```python
from build123d import *

# Parameters (mm, degrees)
CROQUIS1_R                  = 3.1
SALIENTE_EXTRUIR1_DEPTH     = 2.5
CROQUIS2_W                  = 6.5
CROQUIS2_H                  = 10
SALIENTE_EXTRUIR3_DEPTH     = 6
CROQUIS5_W                  = 1.5
CROQUIS5_H                  = 10
CORTAR_EXTRUIR2_DEPTH       = 3
SALIENTE_EXTRUIR4_START     = -3
CROQUIS6_W                  = 5
CROQUIS6_H                  = 10
SALIENTE_EXTRUIR4_DEPTH     = 4
REDONDEO1_R                 = 3
CROQUIS7_W                  = 6.5
CROQUIS7_H                  = 10
SALIENTE_EXTRUIR5_DEPTH     = 3
CHAFL_N1_SIZE2              = 3
CHAFL_N1_SIZE               = 1.732050808
CROQUIS8_W                  = 5
CROQUIS8_H                  = 10
SALIENTE_EXTRUIR6_DEPTH     = 3
CROQUIS9_W                  = 6.5
CROQUIS9_H                  = 10
SALIENTE_EXTRUIR7_DEPTH     = 3
REDONDEO2_R                 = 3
CHAFL_N2_SIZE2              = 3
CHAFL_N2_SIZE               = 1.732050808
REDONDEO1_OF_SIMETR_A1_R    = 3
CHAFL_N1_OF_SIMETR_A1_SIZE2 = 1.732050808
CHAFL_N1_OF_SIMETR_A1_SIZE  = 3
REDONDEO2_OF_SIMETR_A1_R    = 3
CHAFL_N2_OF_SIMETR_A1_SIZE2 = 1.732050808
CHAFL_N2_OF_SIMETR_A1_SIZE  = 3
CROQUIS10_W                 = 10
CROQUIS10_H                 = 6.5
SALIENTE_EXTRUIR9_DEPTH     = 6
CROQUIS12_W                 = 10
CROQUIS12_H                 = 1.5
CORTAR_EXTRUIR6_DEPTH       = 3
CROQUIS13_W                 = 10
CROQUIS13_H                 = 5
SALIENTE_EXTRUIR10_DEPTH    = 3
CROQUIS14_W                 = 10
CROQUIS14_H                 = 6.5
SALIENTE_EXTRUIR11_DEPTH    = 3
REDONDEO3_R                 = 3
CHAFL_N3_SIZE2              = 1.732050808
CHAFL_N3_SIZE               = 3
REDONDEO3_OF_SIMETR_A2_R    = 3
CHAFL_N3_OF_SIMETR_A2_SIZE2 = 3
CHAFL_N3_OF_SIMETR_A2_SIZE  = 1.732050808
SIMETR_A3_START             = 26.922069807
SIMETR_A3_DEPTH             = 10


# Read off the part's stored shape, not the designer's step: Simetría3
with BuildPart() as part:
    # Croquis1 → Saliente-Extruir1 (new body)
    with BuildSketch(Plane.XY):
        with BuildLine():
            Line((32.732069807, -35), (16.823581959, -35))
            Line((16.823581959, -35), (16.823581959, -55))
            Line((16.823581959, -55), (42.732069807, -55))
            ThreePointArc((42.732069807, -55), (56.874205431, -49.142135624), (62.732069807, -35))
            Line((62.732069807, -35), (62.732069807, 35))
            ThreePointArc((62.732069807, 35), (56.874205431, 49.142135624), (42.732069807, 55))
            Line((42.732069807, 55), (18.885856119, 55))
            Line((18.885856119, 55), (18.885856119, 45))
            Line((18.885856119, 45), (-9.114143881, 45))
            Line((-9.114143881, 45), (-9.114143881, 55))
            Line((-9.114143881, 55), (-32.96035757, 55))
            ThreePointArc((-32.96035757, 55), (-47.102493193, 49.142135624), (-52.96035757, 35))
            Line((-52.96035757, 35), (-52.96035757, -35))
            ThreePointArc((-52.96035757, -35), (-47.102493193, -49.142135624), (-32.96035757, -55))
            Line((-32.96035757, -55), (-6.267930193, -55))
            Line((-6.267930193, -55), (-6.267930193, -35))
            Line((-6.267930193, -35), (-22.96035757, -35))
            ThreePointArc((-22.96035757, -35), (-30.031425382, -32.071067812), (-32.96035757, -25))
            Line((-32.96035757, -25), (-32.96035757, 15.854777846))
            ThreePointArc((-32.96035757, 15.854777846), (-29.16035757, 20.3), (-32.96035757, 24.745222154))
            Line((-32.96035757, 24.745222154), (-32.96035757, 25))
            ThreePointArc((-32.96035757, 25), (-30.031425382, 32.071067812), (-22.96035757, 35))
            Line((-22.96035757, 35), (32.732069807, 35))
            ThreePointArc((32.732069807, 35), (39.803137619, 32.071067812), (42.732069807, 25))
            Line((42.732069807, 25), (42.732069807, 24.745222154))
            ThreePointArc((42.732069807, 24.745222154), (38.932069807, 20.3), (42.732069807, 15.854777846))
            Line((42.732069807, 15.854777846), (42.732069807, -25))
            ThreePointArc((42.732069807, -25), (39.803137619, -32.071067812), (32.732069807, -35))
        make_face()
        with Locations((20.823581959, -39.7)):
            Circle(CROQUIS1_R, mode=Mode.SUBTRACT)
        with Locations((-10.267930193, -39.7)):
            Circle(CROQUIS1_R, mode=Mode.SUBTRACT)
        with Locations((43.432069807, 20.3)):
            Circle(CROQUIS1_R, mode=Mode.SUBTRACT)
        with Locations((-33.66035757, 20.3)):
            Circle(CROQUIS1_R, mode=Mode.SUBTRACT)
    extrude(amount=SALIENTE_EXTRUIR1_DEPTH)

    # Croquis2 → Saliente-Extruir3 (add)
    with BuildSketch(Plane(origin=(0, 0, 0), x_dir=(-1, 0, 0), z_dir=(0, 0, -1))):
        with Locations((41.71035757, -20)):
            Rectangle(CROQUIS2_W, CROQUIS2_H)
        with Locations((41.71035757, 20)):
            Rectangle(CROQUIS2_W, CROQUIS2_H)
    saliente_extruir3 = extrude(amount=SALIENTE_EXTRUIR3_DEPTH)

    # Croquis5 → Cortar-Extruir2 (cut)
    with BuildSketch(Plane(origin=(0, 0, 0), x_dir=(-1, 0, 0), z_dir=(0, 0, -1))):
        with Locations((39.21035757, -20)):
            Rectangle(CROQUIS5_W, CROQUIS5_H)
        with Locations((39.21035757, 20)):
            Rectangle(CROQUIS5_W, CROQUIS5_H)
    cortar_extruir2 = extrude(amount=CORTAR_EXTRUIR2_DEPTH, mode=Mode.SUBTRACT)

    # Croquis6 → Saliente-Extruir4 (add)
    with BuildSketch(Plane(origin=(-38.46035757, 25, -6), x_dir=(1, 0, 0), z_dir=(0, 0, 1)).offset(SALIENTE_EXTRUIR4_START)):
        with Locations((-4, -5)):
            Rectangle(CROQUIS6_W, CROQUIS6_H)
    saliente_extruir4 = extrude(amount=SALIENTE_EXTRUIR4_DEPTH)

    # Redondeo1
    redondeo1_edges = [part.edges().sort_by_distance(p)[0] for p in [
        (-44.96035757, 20, 0),
    ]]
    fillet(redondeo1_edges, radius=REDONDEO1_R)

    # Croquis7 → Saliente-Extruir5 (add)
    with BuildSketch(Plane(origin=(0, 0, -9), x_dir=(-1, 0, 0), z_dir=(0, 0, -1))):
        with Locations((41.71035757, 20)):
            Rectangle(CROQUIS7_W, CROQUIS7_H)
    saliente_extruir5 = extrude(amount=SALIENTE_EXTRUIR5_DEPTH)

    # Chaflán1
    chafl_n1_edges = [part.edges().sort_by_distance(p)[0] for p in [
        (-38.46035757, 20, -12),
    ]]
    chafl_n1_side = [part.faces().sort_by_distance(p)[0] for p in [
        (-38.494998586, 20, -12),
    ]]
    chamfer(chafl_n1_edges, length=CHAFL_N1_SIZE - 0.0001, length2=CHAFL_N1_SIZE2 - 0.0001, reference=chafl_n1_side[0])  # a hair under: the kernel refuses the full size

    # Croquis8 → Saliente-Extruir6 (add)
    with BuildSketch(Plane(origin=(0, 0, -6), x_dir=(-1, 0, 0), z_dir=(0, 0, -1))):
        with Locations((42.46035757, -20)):
            Rectangle(CROQUIS8_W, CROQUIS8_H)
    saliente_extruir6 = extrude(amount=SALIENTE_EXTRUIR6_DEPTH)

    # Croquis9 → Saliente-Extruir7 (add)
    with BuildSketch(Plane(origin=(0, 0, -9), x_dir=(-1, 0, 0), z_dir=(0, 0, -1))):
        with Locations((41.71035757, -20)):
            Rectangle(CROQUIS9_W, CROQUIS9_H)
    saliente_extruir7 = extrude(amount=SALIENTE_EXTRUIR7_DEPTH)

    # Redondeo2
    redondeo2_edges = [part.edges().sort_by_distance(p)[0] for p in [
        (-44.96035757, -20, 0),
    ]]
    fillet(redondeo2_edges, radius=REDONDEO2_R)

    # Chaflán2
    chafl_n2_edges = [part.edges().sort_by_distance(p)[0] for p in [
        (-38.46035757, -20, -12),
    ]]
    chafl_n2_side = [part.faces().sort_by_distance(p)[0] for p in [
        (-38.494998586, -20, -12),
    ]]
    chamfer(chafl_n2_edges, length=CHAFL_N2_SIZE - 0.0001, length2=CHAFL_N2_SIZE2 - 0.0001, reference=chafl_n2_side[0])  # a hair under: the kernel refuses the full size

    # Simetría1: Saliente-Extruir3, Cortar-Extruir2, Saliente-Extruir4, Saliente-Extruir5, Saliente-Extruir6, Saliente-Extruir7 across plane
    add(saliente_extruir3.mirror(Plane(origin=(5.277069807, 0, 0), x_dir=(0, 0, 1), z_dir=(1, 0, 0))))
    add(cortar_extruir2.mirror(Plane(origin=(5.277069807, 0, 0), x_dir=(0, 0, 1), z_dir=(1, 0, 0))), mode=Mode.SUBTRACT)
    add(saliente_extruir4.mirror(Plane(origin=(5.277069807, 0, 0), x_dir=(0, 0, 1), z_dir=(1, 0, 0))))
    add(saliente_extruir5.mirror(Plane(origin=(5.277069807, 0, 0), x_dir=(0, 0, 1), z_dir=(1, 0, 0))))
    add(saliente_extruir6.mirror(Plane(origin=(5.277069807, 0, 0), x_dir=(0, 0, 1), z_dir=(1, 0, 0))))
    add(saliente_extruir7.mirror(Plane(origin=(5.277069807, 0, 0), x_dir=(0, 0, 1), z_dir=(1, 0, 0))))

    # Redondeo1 of Simetría1
    redondeo1_of_simetr_a1_edges = [part.edges().sort_by_distance(p)[0] for p in [
        (55.514497184, 20, 0),
    ]]
    fillet(redondeo1_of_simetr_a1_edges, radius=REDONDEO1_OF_SIMETR_A1_R)

    # Chaflán1 of Simetría1
    chafl_n1_of_simetr_a1_edges = [part.edges().sort_by_distance(p)[0] for p in [
        (49.014497184, 20, -12),
    ]]
    chafl_n1_of_simetr_a1_side = [part.faces().sort_by_distance(p)[0] for p in [
        (49.014497184, 20, -11.965358984),
    ]]
    chamfer(chafl_n1_of_simetr_a1_edges, length=CHAFL_N1_OF_SIMETR_A1_SIZE - 0.0001, length2=CHAFL_N1_OF_SIMETR_A1_SIZE2 - 0.0001, reference=chafl_n1_of_simetr_a1_side[0])  # a hair under: the kernel refuses the full size

    # Redondeo2 of Simetría1
    redondeo2_of_simetr_a1_edges = [part.edges().sort_by_distance(p)[0] for p in [
        (55.514497184, -20, 0),
    ]]
    fillet(redondeo2_of_simetr_a1_edges, radius=REDONDEO2_OF_SIMETR_A1_R)

    # Chaflán2 of Simetría1
    chafl_n2_of_simetr_a1_edges = [part.edges().sort_by_distance(p)[0] for p in [
        (49.014497184, -20, -12),
    ]]
    chafl_n2_of_simetr_a1_side = [part.faces().sort_by_distance(p)[0] for p in [
        (49.014497184, -20, -11.965358984),
    ]]
    chamfer(chafl_n2_of_simetr_a1_edges, length=CHAFL_N2_OF_SIMETR_A1_SIZE - 0.0001, length2=CHAFL_N2_OF_SIMETR_A1_SIZE2 - 0.0001, reference=chafl_n2_of_simetr_a1_side[0])  # a hair under: the kernel refuses the full size

    # Croquis10 → Saliente-Extruir9 (add)
    with BuildSketch(Plane(origin=(0, 0, 0), x_dir=(-1, 0, 0), z_dir=(0, 0, -1))):
        with Locations((21.367930193, -46.75)):
            Rectangle(CROQUIS10_W, CROQUIS10_H)
    saliente_extruir9 = extrude(amount=SALIENTE_EXTRUIR9_DEPTH)

    # Croquis12 → Cortar-Extruir6 (cut)
    with BuildSketch(Plane(origin=(0, 0, 0), x_dir=(-1, 0, 0), z_dir=(0, 0, -1))):
        with Locations((21.367930193, -44.25)):
            Rectangle(CROQUIS12_W, CROQUIS12_H)
    cortar_extruir6 = extrude(amount=CORTAR_EXTRUIR6_DEPTH, mode=Mode.SUBTRACT)

    # Croquis13 → Saliente-Extruir10 (add)
    with BuildSketch(Plane(origin=(0, 0, -6), x_dir=(-1, 0, 0), z_dir=(0, 0, -1))):
        with Locations((21.367930193, -47.5)):
            Rectangle(CROQUIS13_W, CROQUIS13_H)
    saliente_extruir10 = extrude(amount=SALIENTE_EXTRUIR10_DEPTH)

    # Croquis14 → Saliente-Extruir11 (add)
    with BuildSketch(Plane(origin=(0, 0, -9), x_dir=(-1, 0, 0), z_dir=(0, 0, -1))):
        with Locations((21.367930193, -46.75)):
            Rectangle(CROQUIS14_W, CROQUIS14_H)
    saliente_extruir11 = extrude(amount=SALIENTE_EXTRUIR11_DEPTH)

    # Redondeo3
    redondeo3_edges = [part.edges().sort_by_distance(p)[0] for p in [
        (-21.367930193, -50, 0),
    ]]
    fillet(redondeo3_edges, radius=REDONDEO3_R)

    # Chaflán3
    chafl_n3_edges = [part.edges().sort_by_distance(p)[0] for p in [
        (-21.367930193, -43.5, -12),
    ]]
    chafl_n3_side = [part.faces().sort_by_distance(p)[0] for p in [
        (-21.367930193, -43.5, -11.965358984),
    ]]
    chamfer(chafl_n3_edges, length=CHAFL_N3_SIZE - 0.0001, length2=CHAFL_N3_SIZE2 - 0.0001, reference=chafl_n3_side[0])  # a hair under: the kernel refuses the full size

    # Simetría2: Saliente-Extruir9, Cortar-Extruir6, Saliente-Extruir10, Saliente-Extruir11 across plane
    add(saliente_extruir9.mirror(Plane.ZX))
    add(cortar_extruir6.mirror(Plane.ZX), mode=Mode.SUBTRACT)
    add(saliente_extruir10.mirror(Plane.ZX))
    add(saliente_extruir11.mirror(Plane.ZX))

    # Redondeo3 of Simetría2
    redondeo3_of_simetr_a2_edges = [part.edges().sort_by_distance(p)[0] for p in [
        (-21.367930193, 50, 0),
    ]]
    fillet(redondeo3_of_simetr_a2_edges, radius=REDONDEO3_OF_SIMETR_A2_R)

    # Chaflán3 of Simetría2
    chafl_n3_of_simetr_a2_edges = [part.edges().sort_by_distance(p)[0] for p in [
        (-21.367930193, 43.5, -12),
    ]]
    chafl_n3_of_simetr_a2_side = [part.faces().sort_by_distance(p)[0] for p in [
        (-21.367930193, 43.534641016, -12),
    ]]
    chamfer(chafl_n3_of_simetr_a2_edges, length=CHAFL_N3_OF_SIMETR_A2_SIZE - 0.0001, length2=CHAFL_N3_OF_SIMETR_A2_SIZE2 - 0.0001, reference=chafl_n3_of_simetr_a2_side[0])  # a hair under: the kernel refuses the full size

    # Simetría3 outline → Simetría3 (add)
    with BuildSketch(Plane.YZ.offset(SIMETR_A3_START)):
        with BuildLine():
            Line((-45, -3), (-45, 0))
            Line((-45, 0), (-53, 0))
            ThreePointArc((-53, 0), (-50.878679656, -0.878679656), (-50, -3))
            Line((-50, -3), (-50, -12))
            Line((-50, -12), (-45.232050808, -12))
            Line((-45.232050808, -12), (-43.5, -9))
            Line((-43.5, -9), (-45, -9))
            Line((-45, -9), (-45, -6))
            Line((-45, -6), (-43.5, -6))
            Line((-43.5, -6), (-43.5, -3))
            Line((-43.5, -3), (-45, -3))
        make_face()
        with BuildLine():
            Line((43.5, -6), (45, -6))
            Line((45, -6), (45, -9))
            Line((45, -9), (43.5, -9))
            Line((43.5, -9), (45.232050808, -12))
            Line((45.232050808, -12), (50, -12))
            Line((50, -12), (50, -3))
            ThreePointArc((50, -3), (50.878679656, -0.878679656), (53, 0))
            Line((53, 0), (45, 0))
            Line((45, 0), (45, -3))
            Line((45, -3), (43.5, -3))
            Line((43.5, -3), (43.5, -6))
        make_face()
    extrude(amount=SIMETR_A3_DEPTH)


solid = part.part
```
Geometry: final body of the model. Coordinates: model frame, mm. A direction names the side the tool comes from. Give positions to 0.01 mm unless a question says otherwise; leave off trailing zeros. Loops run counter-clockwise (first coordinate to the right, second up) from the corner with the lowest first, then second, coordinate; pieces in that order, holes last. Notation, with made-up numbers: (61, -38) -> (95, -38) arc R21 cw to (95, -20) -> close; hole circle Ø6 at (85.25, 37.25). An arc over 180 degrees is marked (long way). Use CSV: the item, a comma, the result in double quotes.
(1) Pull-direction query (Y, two-part tool) for faces 1 (the face through (36.922, 47, -6)), 2 (the face through (32, 43.5, -4)), 3 (the face through (31.852, 44.354, -10.479)), 4 (the face through (-42, -25, -6)); classes: released by +Y, released by -Y, zero draft, split by the parting line, or undercut.
From the geometry:
face 1,"zero draft"
face 2,"undercut"
face 3,"undercut"
face 4,"released by -Y"
(2) Ray query, line 1 along Y through (x, z) = (51, -7.75); line 2 along Z through (x, y) = (-39.5, -20.5); line 3 along X through (y, z) = (-48, -2.5). Return the intervals inside material, ascending. Write a range as [from, to].
From the geometry:
line 1,"[-25, -15], [15, 25]"
line 2,"[-10.8, -9], [-6, -3], [0, 2.5]"
line 3,"[-26.37, -16.37], [26.92, 36.92]"
(3) Cut plane D-D (y = -8.5). Output: boundary loops of the cut face in (x, z), plus the area to 3 significant figures.
From the geometry:
outline,"(-52.96, 0) -> (-32.96, 0) -> (-32.96, 2.5) -> (-52.96, 2.5) -> close; (42.73, 0) -> (62.73, 0) -> (62.73, 2.5) -> (42.73, 2.5) -> close"
area,"100 mm^2"
(4) First-contact query: P1, Ø6, axis at y = -34, z = -3.5, coming from the +X side; P2, Ø3, axis at y = 44, z = -2, coming from the -X side; P3, Ø2.5, axis at x = 31, z = -7.5, coming from the -Y side; P4, Ø1.5, axis at y = -18.5, z = -4.5, coming from the +X side. Flat tips, straight axial feed; report the tip coordinate or a pass-through.
From the geometry:
P1,"through"
P2,"x = -26.37"
P3,"y = -50"
P4,"x = 55.51"
(5) Access query for faces 5 (the face through (32, -43.5, -5)), 6 (the face through (25, -35, 1)), 7 (the face through (-39.96, -20, -1)), 8 (the face through (-39.314, 19.93, -10.479)), 9 (the face through (-21, 45, -7)). Directions: +Z, -Z, +X, -X, +Y, -Y. A direction counts if a zero-diameter tool reaches every point of the face in a straight line with its end or side. Return the directions, or none.
From the geometry:
face 5,"-Z, +X, -X"
face 6,"+Z, -Z"
face 7,"+Y, -Y"
face 8,"-Z, +Y, -Y"
face 9,"+X, -X"
(6) Cut plane C-C (x = 10.5). Output: boundary loops of the cut face in (y, z).
From the geometry:
outline,"(35, 0) -> (45, 0) -> (45, 2.5) -> (35, 2.5) -> close"
(7) Cut plane B-B (y = -39.7). Output: boundary loops of the cut face in (x, z), plus the area to 3 significant figures.
From the geometry:
outline,"(-52.4, 0) -> (-13.37, 0) -> (-13.37, 2.5) -> (-52.4, 2.5) -> close; (-7.17, 0) -> (-6.27, 0) -> (-6.27, 2.5) -> (-7.17, 2.5) -> close; (16.82, 0) -> (17.72, 0) -> (17.72, 2.5) -> (16.82, 2.5) -> close; (23.92, 0) -> (62.17, 0) -> (62.17, 2.5) -> (23.92, 2.5) -> close"
area,"198 mm^2"
